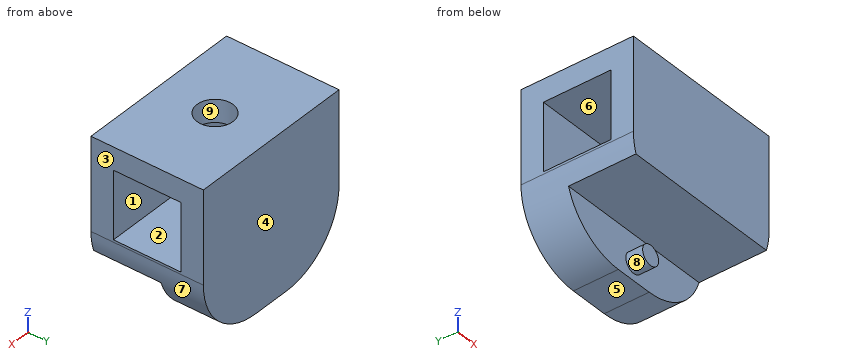
```python
from build123d import *

# Parameters (mm, degrees)
F0_W     = 19.05
F0_H     = 12.7
F1_DEPTH = 6.35
F2_T     = -2.54
F3_R     = 2.032
F4_DEPTH = 2.54
F5_W     = 19.05
F5_H     = 5.08
F6_DEPTH = 5.08
F7_R     = 1.1176
F8_DEPTH = 1.905
F9_R     = 7.358523


with BuildPart() as f1:
    # F0 (on Front) → F1 (new body, symmetric)
    with BuildSketch(Plane.XZ):
        Rectangle(F0_W, F0_H)
    extrude(amount=F1_DEPTH, both=True)

    # F2
    f2_openings = [f1.faces().sort_by_distance(p)[0] for p in [
        (9.525, 0, 0),
        (-9.525, 0, 0),
    ]]
    offset(amount=F2_T, openings=f2_openings)

    # F3 (on face) → F4 (cut)
    with BuildSketch(Plane.XY.offset(6.35)):
        Circle(F3_R)
    extrude(amount=-F4_DEPTH, mode=Mode.SUBTRACT)

    # F5 (on face) → F6 (join)
    with BuildSketch(Plane(origin=(0, 0, -6.35), x_dir=(1, 0, 0), z_dir=(0, 0, -1))):
        with Locations((0, -3.81)):
            Rectangle(F5_W, F5_H)
    extrude(amount=F6_DEPTH)

    # F7 (on face) → F8 (join)
    with BuildSketch(Plane.XZ.offset(-1.27)):
        with Locations((0, -9.525)):
            Circle(F7_R)
    extrude(amount=F8_DEPTH)

    # F9
    f9_edges = [f1.edges().sort_by_distance(p)[0] for p in [
        (9.525, 3.81, -11.43),
        (-9.525, 3.81, -11.43),
    ]]
    fillet(f9_edges, radius=F9_R)


solid = f1.part
```
Build history of the part. All positions in model axes, mm. Face numbers are marked on the shaded views. A direction names the side the tool comes from. Round coordinates to 2 decimals unless told otherwise and drop trailing zeros. Write each loop counter-clockwise with the first axis right and the second up, starting at its lowest first coordinate (ties: lowest second). Pieces come first, ordered by that corner, then holes. Notation, with made-up numbers: (-14, 70.5) - (20, 70.5) arc R20 ccw to (20, 107.5) - close; hole circle Ø5 at (-2, -4). An arc over 180 degrees is marked (long way). Answer as CSV lines item,"result".
Q1. Cut at C-C (x = 7.5). Write the cut outline in (y, z), and give its area (3 significant figures).
Report:
outline,"(-6.35, -6.35) - (1.27, -6.35) - (1.27, -9.14) - (6.35, -9.14) - (6.35, 6.35) - (-6.35, 6.35) - close; hole (-3.81, -3.81) - (3.81, -3.81) - (3.81, 3.81) - (-3.81, 3.81) - close"
area,"117 mm^2"
Q2. Tool access for the marked faces 5, 6, 7, 8 and 9: list every direction of +Z, -Z, +X, -X, +Y, -Y with a clear straight run to the whole face (end or side of a thin tool).
Report:
face 5,"-Z, +X, -X, +Y, -Y"
face 6,"+X, -X"
face 7,"-Z, +X, +Y, -Y"
face 8,"-Y"
face 9,"+Z"
Q3. Cut at A-A (y = 0). Write the cut outline in (x, z) (3 decimals), and give its area (3 significant figures).
Report:
outline,"(-9.525, -4.071) arc R7.359 ccw to (-9.163, -6.35) - (9.163, -6.35) arc R7.359 ccw to (9.525, -4.071) - (9.525, -3.81) - (-9.525, -3.81) - close; (-9.525, 3.81) - (-2.032, 3.81) - (-2.032, 6.35) - (-9.525, 6.35) - close; circle Ø2.235 at (0, -9.525); (2.032, 3.81) - (9.525, 3.81) - (9.525, 6.35) - (2.032, 6.35) - close"
area,"89.8 mm^2"
Q4. Drill centre lines: probe 1 along Z at (x, y) = (-0.75, -3.75); probe 2 along Y at (x, z) = (0, 5.6). Where is each one in solid material? Low to high. Write a range as [from, to].
Report:
probe 1,"z = [-6.35, -3.81], [3.81, 6.35]"
probe 2,"y = [-6.35, -2.03], [2.03, 6.35]"
Q5. Pull direction Y, two halves, no side cores. Call the marked faces 1, 2, 3 and 4: +Y half, -Y half, draft (parallel to the pull), parting line (faces both ways), or undercut.
Report:
face 1,"undercut"
face 2,"undercut"
face 3,"draft"
face 4,"+Y half"
Q6. Cut at B-B (x = 0). Write the cut outline in (y, z) (3 decimals).
Report:
outline,"(-6.35, -6.35) - (1.27, -6.35) - (1.27, -8.407) - (-0.635, -8.407) - (-0.635, -10.643) - (1.27, -10.643) - (1.27, -11.43) - (6.35, -11.43) - (6.35, 6.35) - (2.032, 6.35) - (2.032, 3.81) - (3.81, 3.81) - (3.81, -3.81) - (-3.81, -3.81) - (-3.81, 3.81) - (-2.032, 3.81) - (-2.032, 6.35) - (-6.35, 6.35) - close"
Q7. Cut at D-D (y = 5.5). Write the cut outline in (x, z) (3 decimals).
Report:
outline,"(-9.525, -4.071) arc R7.359 ccw to (-2.166, -11.43) - (2.166, -11.43) arc R7.359 ccw to (9.525, -4.071) - (9.525, 6.35) - (-9.525, 6.35) - close"
Q8. Drop flat-ended pins along their axis: pin 1 (0.7 mm diameter, centred on x = 0, z = -9.5, fed in from -Y) (3 decimals); pin 2 (2 mm diameter, centred on y = 1, z = -8.5, fed in from -X); pin 3 (2.5 mm diameter, centred on x = 3.5, z = -10, fed in from -Y). Give the stop position or say it passes through.
Report:
pin 1,"stops at y = -0.635"
pin 2,"stops at x = -8.66"
pin 3,"stops at y = 1.27"
